from build123d import *

# Parameters (mm, degrees)
EXTRUDE_1_DEPTH     = 25
SKETCH_3_R          = 8
CUT_EXTRUDE_2_DEPTH = 52.565492337


with BuildPart() as part:
    # Эскиз2 → Бобышка-Вытянуть1 (new body)
    with BuildSketch(Plane.XY):
        Polygon((-45, 0), (45, 0), (42.899377385, 3), (-40.71555598, 3), align=None)
    extrude(amount=EXTRUDE_1_DEPTH)

    # Эскиз3 → Вырез-Вытянуть2 (cut, through all)
    with BuildSketch(Plane(origin=(0, 3, 0), x_dir=(1, 0, 0), z_dir=(0, 1, 0))):
        with Locations(Location((-22, -12.5, 0), (0, 0, 180))):
            Circle(SKETCH_3_R)
        with Locations(Location((22, -12.5, 0), (0, 0, 180))):
            Circle(SKETCH_3_R)
    extrude(amount=-CUT_EXTRUDE_2_DEPTH, mode=Mode.SUBTRACT)


solid = part.part
Model file for the job. Use its own axes, mm. Coordinates: 2 decimals unless noted, no trailing zeros. Loops run counter-clockwise (first coordinate to the right, second up) from the corner with the lowest first, then second, coordinate; pieces in that order, holes last. Notation, with made-up numbers: (62.5, -13.75) -> (105.5, -13.75) arc R12 ccw to (105.5, 6.25) -> close; hole circle Ø4 at (-30, -38). An arc over 180 degrees is marked (long way). Use one line per item in the form item = value. Start each with the question number.
(1) Flat gauge pins, fed straight in: pin 1 (14.5 mm diameter, centred on x = 22, z = 12.5, fed in from +Y); pin 2 (1.5 mm diameter, centred on y = 1.5, z = 17, fed in from -X). Where does each tip first touch, or does it go through?
(2) Probe probe 1 along X at (y, z) = (0.6, 13.5); probe 2 along X at (y, z) = (1.05, 11.25); probe 3 along Z at (x, y) = (21.5, 1.5). List the from-to ranges inside material, lowest first. Write a range as from..to.
(3) Pull direction X, two halves, no side cores. Call faces 1 (the cylindrical face through (28.349, 1.521, 7.632)), 2 (the flat face through (-1, 2, 25)), 3 (the flat face through (-42.83, 1.52, 12.32)): pulls with the +X half, pulls with the -X half, needs draft (parallel to the pull), parting line crosses it, or undercut.
(4) Cut at D-D on z = 7.75. Give the cut face in (x, y), and give its area (3 significant figures).
(5) Cut at C-C on y = 0.45. Give the cut face in (x, z), and give its area (3 significant figures).
(6) Cut at A-A on x = 22. Give the cut face in (y, z).
(7) Cut at B-B on z = 12.5. Give the cut face in (x, y), and give its area (3 significant figures).
Values:
q1.pin_1 = through
q1.pin_2 = -43.93
q2.probe_1 = -44.14..-29.94, -14.06..14.06, 29.94..44.58
q2.probe_2 = -43.5..-29.9, -14.1..14.1, 29.9..44.26
q2.probe_3 = 0..4.52, 20.48..25
q3.face_1 = undercut
q3.face_2 = needs draft
q3.face_3 = pulls with the -X half
q4.outline = (-45, 0) -> (-28.44, 0) -> (-28.44, 3) -> (-40.72, 3) -> close; (-15.56, 0) -> (15.56, 0) -> (15.56, 3) -> (-15.56, 3) -> close; (28.44, 0) -> (45, 0) -> (42.9, 3) -> (28.44, 3) -> close
q4.area = 183 mm2
q5.outline = (-44.36, 0) -> (44.68, 0) -> (44.68, 25) -> (-44.36, 25) -> close; hole circle Ø16 at (-22, 12.5); hole circle Ø16 at (22, 12.5)
q5.area = 1,820 mm2
q6.outline = (0, 0) -> (3, 0) -> (3, 4.5) -> (0, 4.5) -> close; (0, 20.5) -> (3, 20.5) -> (3, 25) -> (0, 25) -> close
q7.outline = (-45, 0) -> (-30, 0) -> (-30, 3) -> (-40.72, 3) -> close; (-14, 0) -> (14, 0) -> (14, 3) -> (-14, 3) -> close; (30, 0) -> (45, 0) -> (42.9, 3) -> (30, 3) -> close
q7.area = 164 mm2
